Solid Edge part; units mm, degrees
sketch "Sketch1" plane through (0, 0, 0) normal (0, 0, 1) x (1, 0, 0)
  circle A0 centre (0, 0) radius 18
  circle A1 centre (0, 0) radius 5
  circle A2 centre (8, 0) radius 1.15
  circle A3 centre (0, 8) radius 1.15
  circle A4 centre (-8, 0) radius 1.15
  circle A5 centre (0, -8) radius 1.15
extrude "Protrusion1" add sketch "Sketch1" along normal blind 4
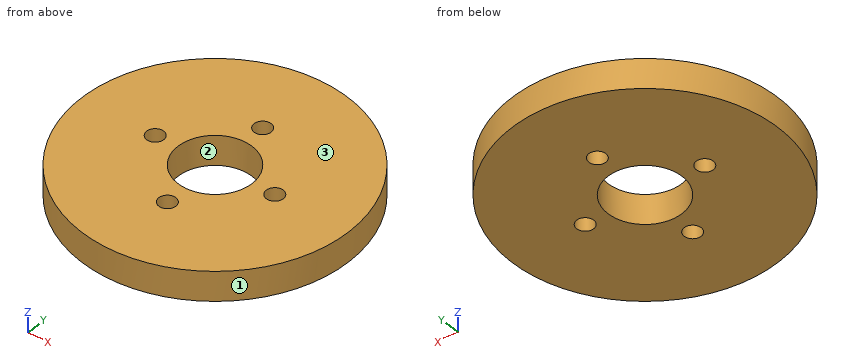
Source: CAD feature listing. Evaluate the final solid. Frame: model axes, mm. Face numbers are marked on the shaded views. Round coordinates to 2 decimals unless told otherwise and drop trailing zeros. Loops run counter-clockwise (first coordinate to the right, second up) from the corner with the lowest first, then second, coordinate; pieces in that order, holes last. Notation, with made-up numbers: M -19.5,-37 L 38.5,-37 A17 cw 38.5,-8 Z; hole C -12,55 d2. An arc over 180 degrees is marked long. Return JSON: item names as keys, results as strings. Group by question number.
1. Mould query, pull axis X, two halves, no side actions, for the marked faces 1, 2 and 3. Classes: released by +X, released by -X, zero draft, split by the parting line, or undercut.
2. Pin query (flat end, axial travel): pin 1 (1.5 mm diameter, centred on y = 12.5, z = 2, fed in from -X); pin 2 (2 mm diameter, centred on y = -3.5, z = 3, fed in from +X); pin 3 (6 mm diameter, centred on x = 0, y = 0, fed in from +Z). Return the tip coordinate at first contact, or that it passes through.
3. Material intervals for line 1 along Y through (x, z) = (-8, 2.55); line 2 along Y through (x, z) = (-15.5, 3.3); line 3 along X through (y, z) = (-3, 0.2), sorted ascending. Write a range as from..to.
4. Section query D-D on x = -8. Output: boundary loops of the cut face in (y, z), and give its area (3 significant figures).
5. Section query A-A on y = 0. Output: boundary loops of the cut face in (x, z).
6. Section query C-C on z = 1.05. Output: boundary loops of the cut face in (x, y).
Checks:
{
 "1": {"face 1": "split by the parting line", "face 2": "undercut", "face 3": "zero draft"},
 "2": {"pin 1": "stops at x = -13.64", "pin 2": "stops at x = 17.83", "pin 3": "passes through"},
 "3": {"line 1": "y = -16.12..-1.15, 1.15..16.12", "line 2": "y = -9.15..9.15", "line 3": "x = -17.75..-4, 4..17.75"},
 "4": {"outline": "M -16.12,0 L -1.15,0 L -1.15,4 L -16.12,4 Z; M 1.15,0 L 16.12,0 L 16.12,4 L 1.15,4 Z", "area": "120 mm²"},
 "5": {"outline": "M -18,0 L -9.15,0 L -9.15,4 L -18,4 Z; M -6.85,0 L -5,0 L -5,4 L -6.85,4 Z; M 5,0 L 6.85,0 L 6.85,4 L 5,4 Z; M 9.15,0 L 18,0 L 18,4 L 9.15,4 Z"},
 "6": {"outline": "C 0,0 d36; hole C -8,0 d2.3; hole C 0,0 d10; hole C 0,-8 d2.3; hole C 0,8 d2.3; hole C 8,0 d2.3"}
}
